```python
from build123d import *

# Parameters (mm, degrees)
F1_DEPTH = 25.4
F3_DEPTH = 25.4
F5_DEPTH = 25.4


with BuildPart() as f1:
    # F0 (on Top) → F1 (new body)
    with BuildSketch(Plane.XY):
        Polygon((-3.807562, -21.711232), (39.454739, -41.670527), (-7.130801, 18.008294), align=None)
        with BuildLine():
            Line((-3.807562, -21.711232), (0, -67.2194))
            ThreePointArc((0, -67.2194), (23.511012, -60.287986), (39.454739, -41.670527))
            Line((39.454739, -41.670527), (-3.807562, -21.711232))
        make_face()
    extrude(amount=F1_DEPTH)

    # F2 (on Top) → F3 (join)
    with BuildSketch(Plane.XY):
        with BuildLine():
            ThreePointArc((-42.670067, -28.083367), (-9.526807, -31.983188), (0, 0))
            ThreePointArc((0, 0), (-27.873553, -4.107011), (-42.670067, -28.083367))
        make_face()
    extrude(amount=F3_DEPTH)

    # F4 (on face) → F5 (cut)
    with BuildSketch(Plane.XY.offset(25.4)):
        Polygon((-9.030846, -5.911056), (-22.315262, -7.504281), (-11.007384, -7.504281), align=None)
        Polygon((-5.722075, -3.243963), (-9.030846, -5.911056), (1.316611, -4.670067), align=None)
        Polygon((-30.981028, -12.238209), (-35.863359, -24.257382), (-30.248286, -30.385217), (-24.002817, -32.40481), (-17.116513, -30.688128), (-9.888924, -28.083367), (0, -20.580618), (1.226096, -25.366375), (7.193933, -62.676668), (20.713773, -58.206778), (29.183986, -49.159691), (34.290549, -40.386488), (10.949366, -10.485058), (1.316611, -4.670067), (-9.030846, -5.911056), (-11.007384, -7.504281), (-22.315262, -7.504281), align=None)
    extrude(amount=-F5_DEPTH, mode=Mode.SUBTRACT)


solid = f1.part
```
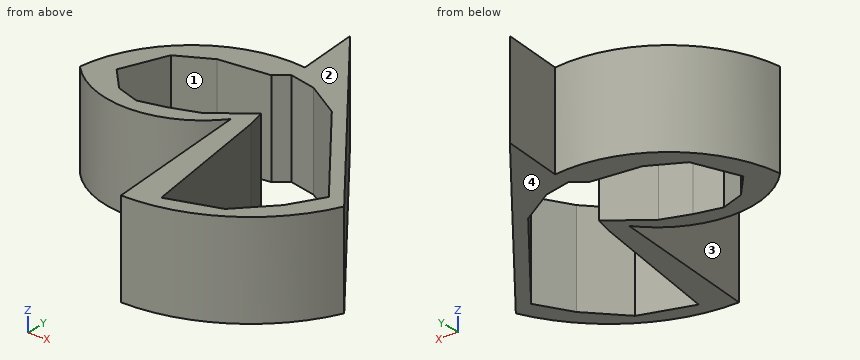
The listing builds one solid part. Answer for the finished solid, in the listing's coordinates (mm). Face numbers are marked on the shaded views. A direction names the side the tool comes from. Give positions to 0.01 mm unless a question says otherwise; leave off trailing zeros. Order: outer loops, then holes, each group sorted by start corner. A loop starts at its lowest first (then second) coordinate and runs counter-clockwise, first axis right, second up. Notation, with made-up numbers: (53.5, -3) -> (76.5, -3) arc R15 cw to (76.5, 19) -> close; hole circle Ø10 at (-23, 13). An arc over 180 degrees is marked (long way). Write each question's results on one line, items separated by ' | '.
Q1. Determine the mould class of the marked faces 3 and 4 for opening direction X: pulls with the +X half, pulls with the -X half, needs draft (parallel to the pull), parting line crosses it, or undercut.
Checked values:
face 3: undercut | face 4: needs draft
Q2. Which of the six approach directions +Z, -Z, +X, -X, +Y, -Y give full straight-line access (tool end or side, diameter ignored) to the marked faces 1 and 2?
Checked values:
face 1: +Z, -Z | face 2: +Z, +X, -X, +Y, -Y
Q3. The part is cut by section A-A, the plane z = 3.75. Give the vertices of the cut face in (x, y) (1 decimal).
Checked values:
outline: (-42.7, -28.1) arc R25.9 ccw to (-3.4, -26.4) -> (0, -67.2) arc R43.2 ccw to (39.5, -41.7) -> (-7.1, 18) -> (-5.7, 1.2) arc R33.4 ccw to start; hole (-35.9, -24.3) -> (-30.2, -30.4) -> (-24, -32.4) -> (-17.1, -30.7) -> (-9.9, -28.1) -> (0, -20.6) -> (1.2, -25.4) -> (7.2, -62.7) -> (20.7, -58.2) -> (29.2, -49.2) -> (34.3, -40.4) -> (10.9, -10.5) -> (1.3, -4.7) -> (-5.7, -3.2) -> (-9, -5.9) -> (-22.3, -7.5) -> (-31, -12.2) -> close
Q4. The part is cut by section B-B, the plane x = 23.5. Give the vertices of the cut face in (y, z).
Checked values:
outline: (-60.3, 0) -> (-55.23, 0) -> (-55.23, 25.4) -> (-60.3, 25.4) -> close; (-26.56, 0) -> (-21.23, 0) -> (-21.23, 25.4) -> (-26.56, 25.4) -> close
Q5. The part is cut by section D-D, the plane y = 7. Give the vertices of the cut face in (x, z).
Checked values:
outline: (-6.21, 0) -> (1.46, 0) -> (1.46, 25.4) -> (-6.21, 25.4) -> close
Q6. The part is cut by section C-C, the plane y = -15. Give the vertices of the cut face in (x, z), and give its area (3 significant figures).
Checked values:
outline: (-38.25, 0) -> (-32.1, 0) -> (-32.1, 25.4) -> (-38.25, 25.4) -> close; (14.47, 0) -> (18.64, 0) -> (18.64, 25.4) -> (14.47, 25.4) -> close | area: 262 mm^2
Q7. Straight lines are drawn through the part: probe 1 along X at (y, z) = (-8, 22.25); probe 2 along Y at (x, z) = (26.5, 5.5); probe 3 along Y at (x, z) = (-29, 19). For each, find the intervals that lie inside material, in ascending order. Write a range as from..to.
Checked values:
probe 1: x = -32.73..-23.22, 6.83..13.17 | probe 2: y = -58.17..-52.03, -30.41..-25.07 | probe 3: y = -35.72..-30.79, -11.16..-4.88
Q8. Each of these flat-tipped pins is pushed along its axis until it touches: P1, Ø4, axis at x = 8, z = 21.5, coming from the -Y side; P2, Ø2, axis at y = -9, z = 3, coming from the -X side; P3, Ø12, axis at y = 3, z = 18.5, coming from the +X side. Where does it stop, or does it pass through?
Checked values:
P1: stops at y = -66.81 | P2: stops at x = -34.64 | P3: stops at x = 9.27
